Part model, mm, in its own coordinate system. Face numbers are marked on the shaded views. A direction names the side the tool comes from. Round coordinates to 2 decimals unless told otherwise and drop trailing zeros. Loops run counter-clockwise (first coordinate to the right, second up) from the corner with the lowest first, then second, coordinate; pieces in that order, holes last. Notation, with made-up numbers: M -27.5,46.25 L 24.5,46.25 A29 cw 24.5,85.25 Z; hole C 76,21.5 d9. An arc over 180 degrees is marked long. Answer as CSV lines item,"result". Start each with the question number.
Item 1: Band-saw the part on D-D (y = -8). Give the cut face in (x, z), and give its area (3 significant figures).
Item 2: Band-saw the part on C-C (z = -10). Give the cut face in (x, y).
Item 3: Band-saw the part on B-B (x = -3). Give the cut face in (y, z), and give its area (3 significant figures).
Item 4: Drop flat-ended pins along their axis: pin 1 Ø4 at (x, z) = (-11, 40) entering from +Y; pin 2 Ø6 at (y, z) = (4, 17) entering from -X; pin 3 Ø8 at (x, z) = (4.5, 72) entering from +Y; pin 4 Ø3 at (x, z) = (11, -2.5) entering from -Y. Give the stop position or say it passes through.
Item 5: Band-saw the part on A-A (z = 2.5). Give the cut face in (x, y).
Item 6: Wall check: line 1 (Y direction, x = 0, z = 2.05); line 2 (Z direction, x = -5, y = 10.5); line 3 (X direction, y = -14, z = 4.55). Give the ranges that are in metal, low to high.
Item 7: Which spindle directions (+Z, -Z, +X, -X, +Y, -Y) get a long thin tool onto all of the face, cutting with end or side? Do the marked faces 1 and 2. Say none if no direction does.
Autodesk Inventor part; units mm, degrees
ref_plane "YZ Plane" through (0, 0, 0) normal (1, 0, 0) x (0, 1, 0)
ref_plane "XZ Plane" through (0, 0, 0) normal (0, 1, 0) x (-1, 0, 0)
ref_plane "XY Plane" through (0, 0, 0) normal (0, 0, 1) x (1, 0, 0)
sketch "Sketch1" plane through (0, 0, 0) normal (0, 0, 1) x (1, 0, 0)
  circle A0 centre (0, 0) radius 19.5
  circle A1 centre (0, 0) radius 4
  dimension "d0" = 39
  dimension "d3" = 8
extrude "Extrusion1" add sketch "Sketch1" along normal blind 90 contours A0 | A1
extrude "Extrusion2" add sketch "Sketch1" against normal blind 20 contours A1
sketch "Sketch2" plane through (0, 0, 0) normal (0, 0, -1) x (-1, 0, 0)
  circle A0 centre (0, 0) radius 4
  circle A1 centre (0, 0) radius 19.5
sketch "Sketch3" plane through (0, 0, 0) normal (0, 0, -1) x (-1, 0, 0)
  circle A0 centre (0, 0) radius 19.5
  circle A1 centre (0, 0) radius 14 construction
  point P0 (14, 0)
  dimension "d6" = 28
hole "Hole1" at (-14, 0, 0) direction (0, 0, 1) diameter 3 depth 6 tip angle 118
pattern_circular "Circular Pattern1" count 4 over 360 about axis through (0, 0, 0) along (0, 0, 1) of "Hole1"
properties part number "PG36M555_Motor_Dummy"
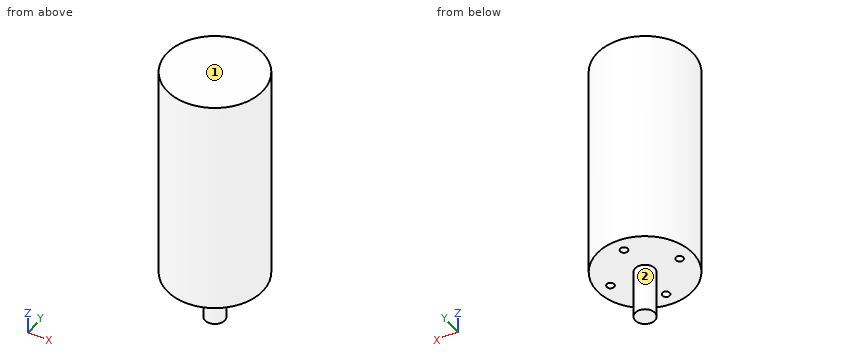
Answer block:
1,outline,"M -17.78,0 L 17.78,0 L 17.78,90 L -17.78,90 Z"
1,area,"3,200 mm^2"
2,outline,"C 0,0 d8"
3,outline,"M -19.27,0 L -2.65,0 L -2.65,-20 L 2.65,-20 L 2.65,0 L 19.27,0 L 19.27,90 L -19.27,90 Z"
3,area,"3,570 mm^2"
4,pin 1,"stops at y = 17.3"
4,pin 2,"stops at x = -19.47"
4,pin 3,"stops at y = 19.49"
4,pin 4,"passes through"
5,outline,"C 0,0 d39; hole C -14,0 d3; hole C 0,-14 d3; hole C 0,14 d3; hole C 14,0 d3"
6,line 1,"y = -19.5 to -15.5, -12.5 to 12.5, 15.5 to 19.5"
6,line 2,"z = 0 to 90"
6,line 3,"x = -13.57 to -1.5, 1.5 to 13.57"
7,face 1,"+Z, +X, -X, +Y, -Y"
7,face 2,"-Z"
